```python
from build123d import *

# Parameters (mm, degrees)
ESBO_O1_W                = 5.9
ESBO_O1_H                = 5.9
RESSALTO_EXTRUS_O1_DEPTH = 3.3
ESBO_O2_R                = 1.65
RESSALTO_EXTRUS_O2_DEPTH = 1


with BuildPart() as part:
    # Esboço1 → Ressalto-extrusão1 (new body)
    with BuildSketch(Plane.XY):
        Rectangle(ESBO_O1_W, ESBO_O1_H)
    extrude(amount=RESSALTO_EXTRUS_O1_DEPTH)

    # Esboço2 → Ressalto-extrusão2 (add)
    with BuildSketch(Plane.XY.offset(3.3)):
        Circle(ESBO_O2_R)
    extrude(amount=RESSALTO_EXTRUS_O2_DEPTH)


solid = part.part
```
Source: CAD feature listing. Evaluate the final solid. Frame: model axes, mm. A direction names the side the tool comes from. Coordinates: 2 decimals unless noted, no trailing zeros. Loops run counter-clockwise (first coordinate to the right, second up) from the corner with the lowest first, then second, coordinate; pieces in that order, holes last. Notation, with made-up numbers: (-28.5, -24) -> (21.5, -24) arc R6 cw to (21.5, -17) -> close; hole circle Ø6 at (-19.5, -2). An arc over 180 degrees is marked (long way). One line per item, written item: value. Start each with the question number.
Q1. Section query D-D, the plane x = -2.1. Return the cut outline in (y, z).
Q2. Line query: line 1 along Z through (x, y) = (0.5, -2.35); line 2 along Y through (x, z) = (-0.6, 3.5); line 3 along X through (y, z) = (0.15, 3.6). Output: solid intervals per line, ascending.
Q3. Section query A-A, the plane x = 0. Return the cut outline in (y, z), and give its area (3 significant figures).
Q4. Section query C-C, the plane z = 3.8. Return the cut outline in (x, y).
Q5. Set-up query: faces 1 (the face through (-1.216, 1.115, 3.793)), 2 (the face through (0, 2.95, 2)). Return all of +Z, -Z, +X, -X, +Y, -Y with unobstructed straight access to the full face (end or side cutting, diameter ignored); none if empty.
Results:
1. outline: (-2.95, 0) -> (2.95, 0) -> (2.95, 3.3) -> (-2.95, 3.3) -> close
2. line 1: 0 to 3.3
2. line 2: -1.54 to 1.54
2. line 3: -1.64 to 1.64
3. outline: (-2.95, 0) -> (2.95, 0) -> (2.95, 3.3) -> (1.65, 3.3) -> (1.65, 4.3) -> (-1.65, 4.3) -> (-1.65, 3.3) -> (-2.95, 3.3) -> close
3. area: 22.8 mm^2
4. outline: circle Ø3.3 at (0, 0)
5. face 1: +Z
5. face 2: +Z, -Z, +X, -X, +Y
